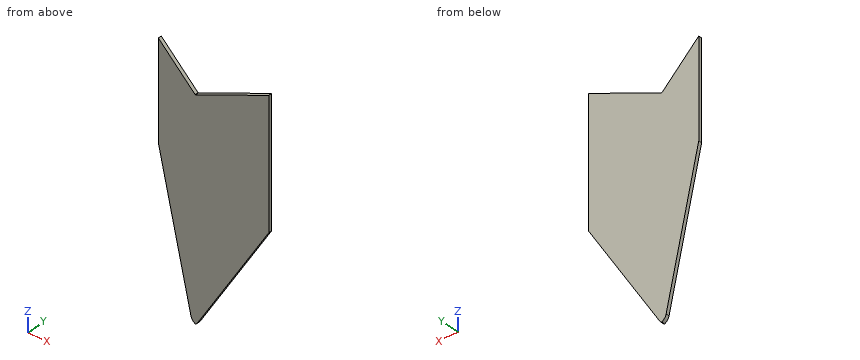
```python
from build123d import *

# Parameters (mm, degrees)
BOSS_EXTRUDE1_DEPTH = 1.27


with BuildPart() as part:
    # Sketch2 → Boss-Extrude1 (new body)
    with BuildSketch(Plane(origin=(0, 0, 0), x_dir=(1, 0, 0), z_dir=(0, 1, 0))):
        with BuildLine():
            Line((-2.543725523, -35.200677289), (-15.887270656, -48.546652053))
            Line((-15.887270656, -48.546652053), (-15.887270656, -12.975156939))
            Line((-15.887270656, -12.975156939), (-4.064387109, 40.624362144))
            ThreePointArc((-4.064387109, 40.624362144), (-3.49318097, 41.819860184), (-2.452860743, 42.640363592))
            ThreePointArc((-2.452860743, 42.640363592), (-2.065756158, 42.410049072), (-1.771451049, 42.069051652))
            Line((-1.771451049, 42.069051652), (24.112729344, -0.05377363))
            Line((24.112729344, -0.05377363), (24.112729344, -46.70931259))
            Line((24.112729344, -46.70931259), (-2.361995962, -35.200677289))
            Line((-2.361995962, -35.200677289), (-2.543725523, -35.200677289))
        make_face()
    extrude(amount=BOSS_EXTRUDE1_DEPTH)


solid = part.part
```
Can you work these out from the model? Positions are in its coordinate system, mm. Round coordinates to 2 decimals unless told otherwise and drop trailing zeros. Loops run counter-clockwise (first coordinate to the right, second up) from the corner with the lowest first, then second, coordinate; pieces in that order, holes last. Notation, with made-up numbers: M -1.5,61.25 L 55.5,61.25 A22 cw 55.5,85.25 Z; hole C -31,52.25 d2. An arc over 180 degrees is marked long. Answer as a JSON object with one key per item and string values. Group by question number.
Q1. Imagine slicing it at D-D, the plane z = -28. Please give me the cut outline in (x, y), then the cut area to 3 significant figures.
Q2. Imagine slicing it at C-C, the plane x = -8. Please give me the cut outline in (y, z).
Q3. Please list where these lines run through material, in increasing order: L1, parallel to Z at x = 15, y = 0.3; L2, parallel to Z at x = 9.5, y = 0.25; L3, parallel to X at y = 1.05, z = 4.5.
Q4. Imagine slicing it at A-A, the plane y = 0.6. Please give me the cut outline in (x, z), then the cut area to 3 significant figures.
Q5. Imagine slicing it at B-B, the plane z = 38. Please give me the cut outline in (x, y).
Findings:
{
 "1": {"outline": "M -6.85,0 L 6.87,0 L 6.87,1.27 L -6.85,1.27 Z", "area": "17.4 mm2"},
 "2": {"outline": "M 0,-22.78 L 1.27,-22.78 L 1.27,40.66 L 0,40.66 Z"},
 "3": {"L1": "z = -14.78 to 42.75", "L2": "z = -23.73 to 40.36", "L3": "x = -14.02 to 24.11"},
 "4": {"outline": "M -15.89,12.98 L -4.06,-40.62 A2.92 ccw -2.45,-42.64 A1.4 ccw -1.77,-42.07 L 24.11,0.05 L 24.11,46.71 L -2.36,35.2 L -2.54,35.2 L -15.89,48.55 Z", "area": "2,450 mm2"},
 "5": {"outline": "M -15.89,0 L -5.34,0 L -5.34,1.27 L -15.89,1.27 Z; M 4.08,0 L 24.11,0 L 24.11,1.27 L 4.08,1.27 Z"}
}
